from build123d import *

# Parameters (mm, degrees)
SKETCH_1_R      = 35
EXTRUDE_1_DEPTH = 2
SKETCH_3_R      = 17.5
EXTRUDE_2_DEPTH = 5
SKETCH_4_R      = 22.5
SKETCH_5_R      = 22.5
EXTRUDE_3_DEPTH = 50
SKETCH_6_R      = 21.322035414
EXTRUDE_4_DEPTH = 50


with BuildPart() as part:
    # 스케치1 → 보스-돌출1 (new body)
    with BuildSketch(Plane.XY):
        Circle(SKETCH_1_R)
    extrude(amount=EXTRUDE_1_DEPTH)

    # 로프트1: read off the stored shape, not the designer's step
    # 로프트1: loft between two sections, ruled curve by curve
    loft_1_from = [
        Edge.make_bspline([(-20.830307169, 8.505780579, 27), (-3.81874601, 50.166394916, 27), (37.841868327, 33.154833758, 27), (20.830307169, -8.505780579, 27), (3.81874601, -50.166394916, 27), (-37.841868327, -33.154833758, 27), (-20.830307169, 8.505780579, 27)], [0, 0, 0, 0, 0.5, 0.5, 0.5, 1, 1, 1, 1], 3, [1, 0.333333333, 0.333333333, 1, 0.333333333, 0.333333333, 1]),
    ]
    loft_1_to = [
        Edge.make_bspline([(10.501396718, 33.38743277, 2), (77.276262258, 12.384639333, 2), (56.273468821, -54.390226207, 2), (-10.501396718, -33.38743277, 2), (-77.276262258, -12.384639333, 2), (-56.273468821, 54.390226207, 2), (10.501396718, 33.38743277, 2)], [0, 0, 0, 0, 0.5, 0.5, 0.5, 1, 1, 1, 1], 3, [1, 0.333333333, 0.333333333, 1, 0.333333333, 0.333333333, 1]),
    ]
    loft_1 = Solid(Shell([*[Face.make_surface_from_curves(loft_1_from[k], loft_1_to[k]) for k in range(1)], Face(Wire(loft_1_from)), Face(Wire(loft_1_to))]))
    add(loft_1)

    # 스케치3 → 보스-돌출2 (add)
    with BuildSketch(Plane.XY.offset(27)):
        Circle(SKETCH_3_R)
    extrude(amount=EXTRUDE_2_DEPTH)

    # 스케치4 → section 0 of loft_2
    with BuildSketch(Plane.XY.offset(42), mode=Mode.PRIVATE) as loft_2_s0:
        Circle(SKETCH_4_R)
    # loft up to a face of the part (loft_2)
    loft([loft_2_s0.sketch, Face(Wire([part.edges().sort_by_distance((-11.979574354, 12.75695098, 32))[0]]))])

    # 스케치5 → 보스-돌출3 (add)
    with BuildSketch(Plane.XY.offset(42)):
        Circle(SKETCH_5_R)
    extrude(amount=EXTRUDE_3_DEPTH)

    # 스케치6 → 보스-돌출4 (add)
    with BuildSketch(Plane.XY.offset(92)):
        Circle(SKETCH_6_R)
    extrude(amount=EXTRUDE_4_DEPTH)


solid = part.part
Source: CAD feature listing. Evaluate the final solid. Frame: model axes, mm. A direction names the side the tool comes from. Round coordinates to 2 decimals unless told otherwise and drop trailing zeros. Loops run counter-clockwise (first coordinate to the right, second up) from the corner with the lowest first, then second, coordinate; pieces in that order, holes last.
Q1. Section A-A, the plane z = 131. Return loops of the section in (x, y), plus the area to 3 significant figures.
Q2. Section B-B, the plane z = 60.5. Return loops of the section in (x, y), plus the area to 3 significant figures.
Q3. Mould query, pull axis Z, two halves, no side actions, for faces 1 (the face through (-13.887, -10.648, 29.465)), 2 (the face through (0, 0, 142)), 3 (the face through (0, 0, 0)), 4 (the face through (-16.9, -13, 116.6)). Classes: pulls with the +Z half, pulls with the -Z half, needs draft (parallel to the pull), parting line crosses it, or undercut.
Q4. First-contact query: P1, Ø8, axis at x = -23.5, y = 27, coming from the +Z side; P2, Ø3, axis at y = 13, z = 63.5, coming from the -X side; P3, Ø1.5, axis at x = -19, z = 80.5, coming from the +Y side. Flat tips, straight axial feed; report the tip coordinate or a pass-through.
Q5. Access query for faces 5 (the face through (8, -20, 92)), 6 (the face through (-14, -11, 27)), 7 (the face through (-28, -21, 1)). Directions: +Z, -Z, +X, -X, +Y, -Y. A direction counts if a zero-diameter tool reaches every point of the face in a straight line with its end or side. Return the directions, or none.
Q6. Ray query, line 1 (Z direction, x = -7, y = -18); line 2 (Z direction, x = -11, y = -23); line 3 (Y direction, x = 3.5, z = 67.5). Return the intervals inside material, ascending.
Solutions:
1. outline: circle Ø42.64 at (0, 0)
1. area: 1,430 mm2
2. outline: circle Ø45 at (0, 0)
2. area: 1,590 mm2
3. face 1: undercut
3. face 2: pulls with the +Z half
3. face 3: pulls with the -Z half
3. face 4: needs draft
4. P1: stops at z = 4.48
4. P2: stops at x = -19.34
4. P3: stops at y = 13.16
5. face 5: +Z
5. face 6: none
5. face 7: +Z, -Z
6. line 1: z = 0 to 27, 35.63 to 142
6. line 2: z = 0 to 9.94
6. line 3: y = -22.23 to 22.23
